from build123d import *

# Parameters (mm, degrees)
BOSS_EXTRUDE2_DEPTH     = 33
CUT_EXTRUDE1_DEPTH      = 123.331516789
CUT_EXTRUDE1_DEPTH_BACK = 123.331516789
CUT_EXTRUDE2_DEPTH      = 123.331516789
CUT_EXTRUDE2_DEPTH_BACK = 123.331516789
SKETCH1_5_R             = 4.5
CUT_EXTRUDE3_DEPTH      = 123.331516789
CUT_EXTRUDE3_DEPTH_BACK = 123.331516789
SKETCH3_W               = 9
SKETCH3_H               = 48
CUT_EXTRUDE4_DEPTH      = 113.040171367
CUT_EXTRUDE4_DEPTH_BACK = 113.040171367
SKETCH4_W               = 18
SKETCH4_H               = 24
CUT_EXTRUDE5_DEPTH      = 104.870111197
CUT_EXTRUDE5_DEPTH_BACK = 104.870111197
SKETCH5_W               = 9
SKETCH5_H               = 30
CUT_EXTRUDE6_DEPTH      = 104.870111197
CUT_EXTRUDE6_DEPTH_BACK = 104.870111197
SKETCH6_W               = 6
SKETCH6_H               = 30
SKETCH6_H_2             = 12
CUT_EXTRUDE7_DEPTH      = 104.870111197
CUT_EXTRUDE7_DEPTH_BACK = 104.870111197
SKETCH7_W               = 3
SKETCH7_H               = 12
CUT_EXTRUDE8_DEPTH      = 104.870111197
CUT_EXTRUDE8_DEPTH_BACK = 104.870111197
SKETCH8_W               = 12
SKETCH8_H               = 24
CUT_EXTRUDE10_REACH     = 124.332
SKETCH9_R               = 3
SKETCH10_W              = 18
SKETCH10_H              = 18
CUT_EXTRUDE11_DEPTH     = 27
SKETCH11_W              = 18
SKETCH11_H              = 8.862227293
CUT_EXTRUDE12_DEPTH     = 27


with BuildPart() as part:
    # Sketch1 → Boss-Extrude2 (new body)
    with BuildSketch(Plane(origin=(0, 0, 0), x_dir=(0, 0, -1), z_dir=(1, 0, 0))):
        with BuildLine():
            Line((0, 0), (30, 0))
            Line((30, 0), (30, -44))
            ThreePointArc((30, -44), (20.627416998, -66.627416998), (-2, -76))
            Line((-2, -76), (-12, -76))
            Line((-12, -76), (-48, -76))
            Line((-48, -76), (-72, -76))
            ThreePointArc((-72, -76), (-84.727922061, -70.727922061), (-90, -58))
            Line((-90, -58), (-90, -30))
            ThreePointArc((-90, -30), (-81, -21.137772707), (-72, -30))
            Line((-72, -30), (-72, -58))
            Line((-72, -58), (-48, -58))
            Line((-48, -58), (-48, -40))
            Line((-48, -40), (0, -40))
            Line((0, -40), (0, 0))
        make_face()
    extrude(amount=-BOSS_EXTRUDE2_DEPTH)

    # Sketch1_4 → Cut-Extrude1 (cut, two sides: drawn at the far end of the back side and taken through both)
    with BuildSketch(Plane(origin=(0, 0, 0), x_dir=(0, 0, -1), z_dir=(1, 0, 0)).offset(-CUT_EXTRUDE1_DEPTH_BACK)):
        with BuildLine():
            Line((16, 0), (14, 0))
            Line((14, 0), (14, -15.05572809))
            ThreePointArc((14, -15.05572809), (15, -33), (16, -15.05572809))
            Line((16, -15.05572809), (16, 0))
        make_face()
    extrude(amount=CUT_EXTRUDE1_DEPTH + CUT_EXTRUDE1_DEPTH_BACK, mode=Mode.SUBTRACT)

    # Sketch1_5 → Cut-Extrude2 (cut, two sides: drawn at the far end of the back side and taken through both)
    with BuildSketch(Plane(origin=(0, 0, 0), x_dir=(0, 0, -1), z_dir=(1, 0, 0)).offset(-CUT_EXTRUDE2_DEPTH_BACK)):
        with Locations((-81, -30.138843618)):
            Circle(SKETCH1_5_R)
    extrude(amount=CUT_EXTRUDE2_DEPTH + CUT_EXTRUDE2_DEPTH_BACK, mode=Mode.SUBTRACT)

    # Sketch3 → Cut-Extrude3 (cut, two sides: drawn at the far end of the back side and taken through both)
    with BuildSketch(Plane(origin=(0, 0, 0), x_dir=(1, 0, 0), z_dir=(0, 1, 0)).offset(-CUT_EXTRUDE3_DEPTH_BACK)):
        with Locations((-28.5, -24)):
            Rectangle(SKETCH3_W, SKETCH3_H)
    extrude(amount=CUT_EXTRUDE3_DEPTH + CUT_EXTRUDE3_DEPTH_BACK, mode=Mode.SUBTRACT)

    # Sketch4 → Cut-Extrude4 (cut, two sides: drawn at the far end of the back side and taken through both)
    with BuildSketch(Plane(origin=(0, -58, 0), x_dir=(1, 0, 0), z_dir=(0, 1, 0)).offset(-CUT_EXTRUDE4_DEPTH_BACK)):
        with Locations((-24, -60)):
            Rectangle(SKETCH4_W, SKETCH4_H)
    extrude(amount=CUT_EXTRUDE4_DEPTH + CUT_EXTRUDE4_DEPTH_BACK, mode=Mode.SUBTRACT)

    # Sketch5 → Cut-Extrude5 (cut, two sides: drawn at the far end of the back side and taken through both)
    with BuildSketch(Plane(origin=(0, -40, 0), x_dir=(1, 0, 0), z_dir=(0, 1, 0)).offset(-CUT_EXTRUDE5_DEPTH_BACK)):
        with Locations((-28.5, 15)):
            Rectangle(SKETCH5_W, SKETCH5_H)
    extrude(amount=CUT_EXTRUDE5_DEPTH + CUT_EXTRUDE5_DEPTH_BACK, mode=Mode.SUBTRACT)

    # Sketch6 → Cut-Extrude6 (cut, two sides: drawn at the far end of the back side and taken through both)
    with BuildSketch(Plane(origin=(0, -40, 0), x_dir=(1, 0, 0), z_dir=(0, 1, 0)).offset(-CUT_EXTRUDE6_DEPTH_BACK)):
        with Locations((-21, 15)):
            Rectangle(SKETCH6_W, SKETCH6_H)
        with Locations((-21, -6)):
            Rectangle(SKETCH6_W, SKETCH6_H_2)
    extrude(amount=CUT_EXTRUDE6_DEPTH + CUT_EXTRUDE6_DEPTH_BACK, mode=Mode.SUBTRACT)

    # Sketch7 → Cut-Extrude7 (cut, two sides: drawn at the far end of the back side and taken through both)
    with BuildSketch(Plane(origin=(0, -40, 0), x_dir=(1, 0, 0), z_dir=(0, 1, 0)).offset(-CUT_EXTRUDE7_DEPTH_BACK)):
        Polygon((0, 0), (0, -12), (10.713453575, -12), (10.713453575, 35.251215896), (-3, 35.251215896), (-3, 0), align=None)
        with Locations((-1.5, -6)):
            Rectangle(SKETCH7_W, SKETCH7_H)
    extrude(amount=CUT_EXTRUDE7_DEPTH + CUT_EXTRUDE7_DEPTH_BACK, mode=Mode.SUBTRACT)

    # Sketch8 → Cut-Extrude8 (cut, two sides: drawn at the far end of the back side and taken through both)
    with BuildSketch(Plane(origin=(0, -40, 0), x_dir=(1, 0, 0), z_dir=(0, 1, 0)).offset(-CUT_EXTRUDE8_DEPTH_BACK)):
        with Locations((-12, -30)):
            Rectangle(SKETCH8_W, SKETCH8_H)
    extrude(amount=CUT_EXTRUDE8_DEPTH + CUT_EXTRUDE8_DEPTH_BACK, mode=Mode.SUBTRACT)

    # Sketch9 → Cut-Extrude10 (cut, up to next)
    with BuildSketch(Plane.XY, mode=Mode.PRIVATE) as cut_extrude10_sk1:
        with Locations((-10.5, -6)):
            Circle(SKETCH9_R)
    cut_extrude10_tool1 = extrude(cut_extrude10_sk1.sketch, amount=-CUT_EXTRUDE10_REACH, mode=Mode.PRIVATE) & part.part
    add(cut_extrude10_tool1.solids().sort_by_distance((-10.5, -6, 0))[0], mode=Mode.SUBTRACT)

    # Sketch10 → Cut-Extrude11 (cut)
    with BuildSketch(Plane.XY.offset(90)):
        with Locations((-24, -67)):
            Rectangle(SKETCH10_W, SKETCH10_H)
        Polygon((-15, -58), (-33, -42), (-33, -58), align=None)
    extrude(amount=-CUT_EXTRUDE11_DEPTH, mode=Mode.SUBTRACT)

    # Sketch11 → Cut-Extrude12 (cut)
    with BuildSketch(Plane.XY.offset(90)):
        with Locations((-9, -25.568886354)):
            Rectangle(SKETCH11_W, SKETCH11_H)
        Polygon((0, -30), (-18, -30), (-18, -39), (0, -55), align=None)
    extrude(amount=-CUT_EXTRUDE12_DEPTH, mode=Mode.SUBTRACT)


solid = part.part
The listing builds one solid part. Answer for the finished solid, in the listing's coordinates (mm). A direction names the side the tool comes from. Give positions to 0.01 mm unless a question says otherwise; leave off trailing zeros. Write each loop counter-clockwise with the first axis right and the second up, starting at its lowest first coordinate (ties: lowest second). Pieces come first, ordered by that corner, then holes. Notation, with made-up numbers: (74.25, 36) -> (105.25, 36) arc R18 cw to (105.25, 49) -> close; hole circle Ø5 at (55, -5.75). An arc over 180 degrees is marked (long way). Use a Markdown table: item, result.
(1) Section D-D, the plane x = -10.5 is taken. Determine the outline of the cut face in (y, z).
Return value:
| item | result |
|---|---|
| outline | (-76, 2) arc R32 ccw to (-44, -30) -> (0, -30) -> (0, -16) -> (-15.06, -16) arc R9 cw (long way) to (-15.06, -14) -> (-9, -14) -> (-9, 0) -> (-40, 0) -> (-40, 18) -> (-76, 18) -> close; (-76, 42) -> (-40, 42) -> (-40, 48) -> (-58, 48) -> (-58, 72) -> (-45.67, 72) -> (-45.67, 90) -> (-58, 90) arc R18 ccw to (-76, 72) -> close; (-3, -14) -> (0, -14) -> (0, 0) -> (-3, 0) -> close |
(2) Section A-A, the plane z = 24 is taken. Determine the outline of the cut face in (x, y), then the cut area to 3 significant figures.
Return value:
| item | result |
|---|---|
| outline | (-24, -76) -> (-18, -76) -> (-18, -40) -> (-24, -40) -> close; (-6, -76) -> (0, -76) -> (0, -40) -> (-6, -40) -> close |
| area | 432 mm2 |
(3) Find the intervals of material crossed by probe 1 along Y at (x, z) = (-10.5, -6.75); probe 2 along X at (y, z) = (-69, 23); probe 3 along Z at (x, y) = (-19, -40.5), in increasing order. Write a range as from..to.
Return value:
| item | result |
|---|---|
| probe 1 | -74.78..-27.6, -20.4..-9, -3..0 |
| probe 2 | -24..-18, -6..0 |
| probe 3 | 12..48, 72..90 |
(4) Determine the mould class of faces 4 (the cylindrical face through (-25.61, -32.88, 84.57)), 5 (the flat face through (-24, -50, 81)), 6 (the flat face through (-18, -58, 30)), 7 (the cylindrical face through (-11, -33, -15)) for opening direction Y: released by +Y, released by -Y, zero draft, split by the parting line, or undercut.
Return value:
| item | result |
|---|---|
| face 4 | undercut |
| face 5 | released by -Y |
| face 6 | zero draft |
| face 7 | undercut |
(5) Flat-ended cylindrical pins translate along their axes: P1, Ø7, axis at y = -61, z = 30.5, coming from the +X side; P2, Ø2.5, axis at x = -1.5, y = -55, coming from the -Z side; P3, Ø13, axis at x = -13.5, y = -58.5, coming from the -Z side; P4, Ø3, axis at y = -63.5, z = 62.5, coming from the -X side. Find the tip coordinate at first contact, or state that the pin passes through.
Return value:
| item | result |
|---|---|
| P1 | x = 0 |
| P2 | z = 12 |
| P3 | z = -28.98 |
| P4 | x = -15 |
(6) For faces 1 (the flat face through (-12, -58, 42)), 2 (the cylindrical face through (-12.71, -3.97, -6.9)), 3 (the flat face through (-3, -39, -9)), determine the directions among +Z, -Z, +X, -X, +Y, -Y from which every point of the face is accessible in a straight line to the end or side of a thin tool.
Return value:
| item | result |
|---|---|
| face 1 | +Y, -Y |
| face 2 | +Z |
| face 3 | -Z, +X, +Y, -Y |
(7) Section C-C, the plane y = -49 is taken. Determine the outline of the cut face in (x, z) (3 decimals).
Return value:
| item | result |
|---|---|
| outline | (-25.125, 72) -> (-6.75, 72) -> (-6.75, 90) -> (-25.125, 90) -> close; (-24, 12) -> (-18, 12) -> (-18, -29.607) -> (-3, -29.607) -> (-3, 12) -> (0, 12) -> (0, 48) -> (-24, 48) -> close; hole (-18, 18) -> (-6, 18) -> (-6, 42) -> (-18, 42) -> close |
(8) Section B-B, the plane x = -20 is taken. Determine the outline of the cut face in (y, z), then the cut area to 3 significant figures.
Return value:
| item | result |
|---|---|
| outline | (-76, 12) -> (-40, 12) -> (-40, 48) -> (-76, 48) -> close; (-53.56, 72) -> (-30, 72) arc R9 ccw to (-30, 90) -> (-53.56, 90) -> close; hole circle Ø9 at (-30.14, 81) |
| area | 1,780 mm2 |
